Here's how the part is built. I have some questions about the finished solid (model axes, mm). A direction names the side the tool comes from. Round coordinates to 2 decimals unless told otherwise and drop trailing zeros. Order: outer loops, then holes, each group sorted by start corner. A loop starts at its lowest first (then second) coordinate and runs counter-clockwise, first axis right, second up. Notation, with made-up numbers: M -38.5,54.5 L -23.5,54.5 A20 cw -23.5,72.5 Z; hole C 56.25,-37.5 d4. An arc over 180 degrees is marked long. Answer as CSV lines item,"result". Start each with the question number.
```python
from build123d import *

# Parameters (mm, degrees)
BOSS_EXTRUDE1_DEPTH = 35
CUT_EXTRUDE1_REACH  = 42.927
SKETCH3_R           = 1.2
CUT_EXTRUDE2_REACH  = 43.533
SKETCH4_R           = 1.5
CUT_EXTRUDE4_REACH  = 45.012


with BuildPart() as part:
    # Sketch1 → Boss-Extrude1 (new body)
    with BuildSketch(Plane.XY):
        Polygon((0, 0), (0, 20), (15, 20), (15, 15), (5, 15), (5, 0), align=None)
    extrude(amount=BOSS_EXTRUDE1_DEPTH)

    # Sketch3 → Cut-Extrude1 (cut, up to next)
    with BuildSketch(Plane.XZ.offset(-15), mode=Mode.PRIVATE) as cut_extrude1_sk1:
        with Locations((7.692388155, 26.692388155)):
            Circle(SKETCH3_R)
    cut_extrude1_tool1 = extrude(cut_extrude1_sk1.sketch, amount=-CUT_EXTRUDE1_REACH, mode=Mode.PRIVATE) & part.part
    # Sketch3 → Cut-Extrude1 (cut, up to next)
    with BuildSketch(Plane.XZ.offset(-15), mode=Mode.PRIVATE) as cut_extrude1_sk2:
        with Locations((7.692388155, 8.307611845)):
            Circle(SKETCH3_R)
    cut_extrude1_tool2 = extrude(cut_extrude1_sk2.sketch, amount=-CUT_EXTRUDE1_REACH, mode=Mode.PRIVATE) & part.part
    add(cut_extrude1_tool1.solids().sort_by_distance((7.692388, 15, 26.692388))[0], mode=Mode.SUBTRACT)
    add(cut_extrude1_tool2.solids().sort_by_distance((7.692388, 15, 8.307612))[0], mode=Mode.SUBTRACT)

    # Sketch4 → Cut-Extrude2 (cut, up to next)
    with BuildSketch(Plane(origin=(5, 0, 0), x_dir=(0, 0, -1), z_dir=(1, 0, 0)), mode=Mode.PRIVATE) as cut_extrude2_sk1:
        with Locations(Location((-22.5, 8, 0), (0, 0, 90))):
            Circle(SKETCH4_R)
    cut_extrude2_tool1 = extrude(cut_extrude2_sk1.sketch, amount=-CUT_EXTRUDE2_REACH, mode=Mode.PRIVATE) & part.part
    # Sketch4 → Cut-Extrude2 (cut, up to next)
    with BuildSketch(Plane(origin=(5, 0, 0), x_dir=(0, 0, -1), z_dir=(1, 0, 0)), mode=Mode.PRIVATE) as cut_extrude2_sk2:
        with Locations(Location((-12.5, 8, 0), (0, 0, 90))):
            Circle(SKETCH4_R)
    cut_extrude2_tool2 = extrude(cut_extrude2_sk2.sketch, amount=-CUT_EXTRUDE2_REACH, mode=Mode.PRIVATE) & part.part
    add(cut_extrude2_tool1.solids().sort_by_distance((5, 8, 22.5))[0], mode=Mode.SUBTRACT)
    add(cut_extrude2_tool2.solids().sort_by_distance((5, 8, 12.5))[0], mode=Mode.SUBTRACT)

    # Sketch6 → Cut-Extrude4 (cut, up to next)
    with BuildSketch(Plane(origin=(0, 20, 0), x_dir=(1, 0, 0), z_dir=(0, 1, 0)), mode=Mode.PRIVATE) as cut_extrude4_sk1:
        with BuildLine():
            Line((-1.5, -34.5), (-1.5, -42.5))
            ThreePointArc((-1.5, -42.5), (16.17766953, -35.17766953), (23.5, -17.5))
            Line((23.5, -17.5), (15.5, -17.5))
            ThreePointArc((15.5, -17.5), (10.52081528, -29.52081528), (-1.5, -34.5))
        make_face()
    cut_extrude4_tool1 = extrude(cut_extrude4_sk1.sketch, amount=-CUT_EXTRUDE4_REACH, mode=Mode.PRIVATE) & part.part
    add(cut_extrude4_tool1.solids().sort_by_distance((12.030696, 20, 31.030696))[0], mode=Mode.SUBTRACT)


solid = part.part
```
Item 1: Which directions (+Z, -Z, +X, -X, +Y, -Y) give clear straight access to the entire face, cutting with the end or side of a thin tool? Please do faces 4 (the cylindrical face through (7.536, 17.465, 27.882)), 5 (the flat face through (5, 8, 16)).
Item 2: If we section it at C-C on x = 7.25: Please give me the cut outline in (y, z), and give its area (3 significant figures).
Item 3: We'd pull the mould along Y, two halves only. Please class faces 1 (the flat face through (0, 10, 17)), 2 (the cylindrical face through (3, 8, 24)), 3 (the flat face through (7, 20, 17)): pulls with the +Y half, pulls with the -Y half, needs draft (parallel to the pull), parting line crosses it, or undercut.
Item 4: If we section it at D-D on z = 22.5: Please give me the cut outline in (x, y).
Item 5: For P1, Ø4, axis at y = 8, z = 22.5, coming from the +X side; P2, Ø5, axis at x = 10, z = 17, coming from the -Y side, each with a flat end and sliding along its axis, tell me the tip position at first contact or that it passes through.
Item 6: If we section it at B-B on y = 8: Please give me the cut outline in (x, z), and give its area (3 significant figures).
Item 7: If we section it at A-A on z = 12.5: Please give me the cut outline in (x, y).
Item 8: If I drill on line 1 along Z through (x, y) = (1.2, 8); line 2 along Z through (x, y) = (6.75, 16.75); line 3 along X through (y, z) = (4.5, 11.5), over which ranges is the centre line in solid material (lowest first)?
Geometry says:
1,face 4,"+Y, -Y"
1,face 5,"+Z, -Z, +X, -Y"
2,outline,"M 15,0 L 20,0 L 20,7.19 L 15,7.19 Z; M 15,9.42 L 20,9.42 L 20,25.58 L 15,25.58 Z; M 15,27.81 L 20,27.81 L 20,32.08 L 15,32.08 Z"
2,area,"138 mm²"
3,face 1,"needs draft"
3,face 2,"undercut"
3,face 3,"pulls with the +Y half"
4,outline,"M 0,0 L 5,0 L 5,6.5 L 0,6.5 Z; M 0,9.5 L 5,9.5 L 5,15 L 14.75,15 L 14.75,20 L 0,20 Z"
5,P1,"x = 5"
5,P2,"y = 15"
6,outline,"M 0,0 L 5,0 L 5,11 L 0,11 Z; M 0,14 L 5,14 L 5,21 L 0,21 Z; M 0,24 L 5,24 L 5,33.21 A17 ccw 0,34.43 Z"
6,area,"140 mm²"
7,outline,"M 0,0 L 5,0 L 5,6.5 L 0,6.5 Z; M 0,9.5 L 5,9.5 L 5,15 L 15,15 L 15,20 L 0,20 Z"
8,line 1,"0 to 11, 14 to 21, 24 to 34.28"
8,line 2,"0 to 7.56, 9.05 to 25.95, 27.44 to 32.36"
8,line 3,"0 to 5"
